from build123d import *

# Parameters (mm, degrees)
SKETCH1_R                       = 20
SKETCH1_R_2                     = 2.1
SKETCH1_R_3                     = 2.65
SKETCH1_R_4                     = 10
BOSS_EXTRUDE1_DEPTH             = 20
SKIZZE1_R                       = 10
SCHNITT_LINEAR_AUSTRAGEN1_DEPTH = 8


with BuildPart() as part:
    # Sketch1 → Boss-Extrude1 (new body)
    # profile 1 of 2: a face of its own
    with BuildSketch(Plane.XY):
        Circle(SKETCH1_R)
        with Locations((11.136931804, 11.136931804)):
            Circle(SKETCH1_R_2, mode=Mode.SUBTRACT)
        with Locations((-15.75, 0)):
            Circle(SKETCH1_R_3, mode=Mode.SUBTRACT)
        with Locations((0, -15.75)):
            Circle(SKETCH1_R_3, mode=Mode.SUBTRACT)
        with Locations((15.75, 0)):
            Circle(SKETCH1_R_3, mode=Mode.SUBTRACT)
        with Locations((0, 15.75)):
            Circle(SKETCH1_R_3, mode=Mode.SUBTRACT)
        Circle(SKETCH1_R_4, mode=Mode.SUBTRACT)
    # profile 2 of 2: a face of its own
    with BuildSketch(Plane.XY):
        Circle(SKETCH1_R_4)
        with BuildLine():
            Line((5.25, -1.5), (3.761980861, -1.5))
            ThreePointArc((3.761980861, -1.5), (-4.05, 0), (3.761980861, 1.5))
            Line((3.761980861, 1.5), (5.25, 1.5))
            Line((5.25, 1.5), (5.25, -1.5))
        make_face(mode=Mode.SUBTRACT)
    extrude(amount=BOSS_EXTRUDE1_DEPTH)

    # Skizze1 → Schnitt-Linear austragen1 (cut)
    with BuildSketch(Plane(origin=(0, 0, 0), x_dir=(-1, 0, 0), z_dir=(0, 0, -1))):
        Circle(SKIZZE1_R)
    extrude(amount=-SCHNITT_LINEAR_AUSTRAGEN1_DEPTH, mode=Mode.SUBTRACT)


solid = part.part
CAD build for the part. Positions are in the model's coordinates, mm. A direction names the side the tool comes from. Coordinates: 2 decimals unless noted, no trailing zeros. Loops run counter-clockwise (first coordinate to the right, second up) from the corner with the lowest first, then second, coordinate; pieces in that order, holes last. Notation, with made-up numbers: (3.25, 38.25) - (15.25, 38.25) arc R18 ccw to (15.25, 47.25) - close; hole circle Ø11 at (78, 32.5). An arc over 180 degrees is marked (long way). Write item = value, one per line. Start each with the question number.
Q1. Cut at D-D, the plane z = 5.75. List the corners of the cut face in (x, y), then the cut area to 3 significant figures.
Q2. Drill centre lines: L1, parallel to Y at x = 0, z = 15.5; L2, parallel to Y at x = 0, z = 5; L3, parallel to Z at x = -7, y = 0. Where is each one in solid material? Low to high.
Q3. Cut at A-A, the plane y = 0. List the corners of the cut face in (x, z), then the cut area to 3 significant figures.
Q4. Cut at C-C, the plane y = -15.75. List the corners of the cut face in (x, z).
Q5. Pull direction X, two halves, no side cores. Call faces 4 (the flat face through (-4.3, 0.1, 8)), 5 (the cylindrical face through (-4.336, -19.524, 9.86)), 6 (the flat face through (-0.3, -4.2, 20)): pulls with the +X half, pulls with the -X half, needs draft (parallel to the pull), parting line crosses it, or undercut.
Q6. Flat gauge pins, fed straight in: pin 1 Ø3.5 at (x, y) = (11.14, 11.14) entering from -Z; pin 2 Ø6 at (y, z) = (11, 9) entering from -X; pin 3 Ø6 at (x, z) = (-6, 13.5) entering from +Y; pin 4 Ø6 at (x, y) = (3.5, -4.5) entering from -Z. Where does each tip first touch, or does it go through?
Q7. Cut at B-B, the plane x = 0. List the corners of the cut face in (y, z), then the cut area to 3 significant figures.
Q8. Which spindle directions (+Z, -Z, +X, -X, +Y, -Y) get a long thin tool onto all of the face, cutting with end or side? Do faces 1 (the cylindrical face through (2.17, -9.76, 3.94)), 2 (the flat face through (5.25, 0, 14)), 3 (the flat face through (-5, 9, 0)). Say none if no direction does.
Computed:
q1.outline = circle Ø40 at (0, 0); hole circle Ø5.3 at (-15.75, 0); hole circle Ø20 at (0, 0); hole circle Ø5.3 at (0, -15.75); hole circle Ø5.3 at (0, 15.75); hole circle Ø4.2 at (11.14, 11.14); hole circle Ø5.3 at (15.75, 0)
q1.area = 840 mm²
q2.L1 = -20 to -18.4, -13.1 to -4.05, 4.05 to 13.1, 18.4 to 20
q2.L2 = -20 to -18.4, -13.1 to -10, 10 to 13.1, 18.4 to 20
q2.L3 = 8 to 20
q3.outline = (-20, 0) - (-18.4, 0) - (-18.4, 20) - (-20, 20) - close; (-13.1, 0) - (-10, 0) - (-10, 8) - (-4.05, 8) - (-4.05, 20) - (-13.1, 20) - close; (5.25, 8) - (10, 8) - (10, 0) - (13.1, 0) - (13.1, 20) - (5.25, 20) - close; (18.4, 0) - (20, 0) - (20, 20) - (18.4, 20) - close
q3.area = 316 mm²
q4.outline = (-12.33, 0) - (-2.65, 0) - (-2.65, 20) - (-12.33, 20) - close; (2.65, 0) - (12.33, 0) - (12.33, 20) - (2.65, 20) - close
q5.face_4 = undercut
q5.face_5 = parting line crosses it
q5.face_6 = needs draft
q6.pin_1 = through
q6.pin_2 = -18.33
q6.pin_3 = 19.77
q6.pin_4 = 8
q7.outline = (-20, 0) - (-18.4, 0) - (-18.4, 20) - (-20, 20) - close; (-13.1, 0) - (-10, 0) - (-10, 8) - (-4.05, 8) - (-4.05, 20) - (-13.1, 20) - close; (4.05, 8) - (10, 8) - (10, 0) - (13.1, 0) - (13.1, 20) - (4.05, 20) - close; (18.4, 0) - (20, 0) - (20, 20) - (18.4, 20) - close
q7.area = 331 mm²
q8.face_1 = -Z
q8.face_2 = +Z, -Z
q8.face_3 = -Z, +X, -X, +Y, -Y
